from build123d import *

# Parameters (mm, degrees)
SKETCH_1_W               = 80
SKETCH_1_H               = 40
EXTRUDE_1_DEPTH          = 500
EXTRUDE_1_2_DEPTH        = 500
SKETCH_2_W               = 340
SKETCH_2_H               = 40
EXTRUDE_2_DEPTH          = 40
SKETCH_3_W               = 340
SKETCH_3_H               = 40
EXTRUDE_3_DEPTH          = 40
CUT_EXTRUDE_1_DEPTH      = 1
CUT_EXTRUDE_1_DEPTH_BACK = 161
SKETCH_5_W               = 40
SKETCH_5_H               = 200
EXTRUDE_4_DEPTH          = 40
SKETCH_6_W               = 40
SKETCH_6_H               = 200
EXTRUDE_5_DEPTH          = 40


with BuildPart() as part:
    # Sketch 1 → Extrude 1 (new body)
    with BuildSketch(Plane(origin=(0, 0, 0), x_dir=(1, 0, 0), z_dir=(0, 1, 0))):
        with Locations((40, -20)):
            Rectangle(SKETCH_1_W, SKETCH_1_H)
    extrude(amount=EXTRUDE_1_DEPTH)



with BuildPart() as body_2:
    # Sketch 1 → Extrude 1 2 (new body)
    with BuildSketch(Plane(origin=(0, 0, 0), x_dir=(1, 0, 0), z_dir=(0, 1, 0))):
        with Locations((40, 80)):
            Rectangle(SKETCH_1_W, SKETCH_1_H)
    extrude(amount=EXTRUDE_1_2_DEPTH)


with BuildPart() as part_1:
    add(part.part)

    add(body_2.part)  # Extrude 2 merges body 2
    # Sketch 2 → Extrude 2 (add)
    with BuildSketch(Plane(origin=(80, 0, 0), x_dir=(0, 0, -1), z_dir=(1, 0, 0))):
        with Locations((30, 480)):
            Rectangle(SKETCH_2_W, SKETCH_2_H)
    extrude(amount=EXTRUDE_2_DEPTH)

    # Sketch 3 → Extrude 3 (add)
    with BuildSketch(Plane.ZY):
        with Locations((-30, 480)):
            Rectangle(SKETCH_3_W, SKETCH_3_H)
    extrude(amount=EXTRUDE_3_DEPTH)

    # Sketch 4 → Cut-Extrude 1 (cut, two sides)
    with BuildSketch(Plane.ZY.offset(40)) as cut_extrude_1_sk:
        Polygon((140, 460), (100, 500), (140, 500), align=None)
        Polygon((-200, 460), (-160, 500), (-200, 500), align=None)
    extrude(amount=CUT_EXTRUDE_1_DEPTH, mode=Mode.SUBTRACT)
    extrude(cut_extrude_1_sk.sketch, amount=-CUT_EXTRUDE_1_DEPTH_BACK, mode=Mode.SUBTRACT)

    # Sketch 5 → Extrude 4 (add)
    with BuildSketch(Plane(origin=(0, 300, 300), x_dir=(1, 0, 0), z_dir=(0, 0.707106781, 0.707106781))):
        with Locations((-20, 222.842712475)):
            Rectangle(SKETCH_5_W, SKETCH_5_H)
        with Locations((100, 222.842712475)):
            Rectangle(SKETCH_5_W, SKETCH_5_H)
    extrude(amount=EXTRUDE_4_DEPTH)

    # Sketch 6 → Extrude 5 (add)
    with BuildSketch(Plane(origin=(0, 330, -330), x_dir=(1, 0, 0), z_dir=(0, 0.707106781, -0.707106781))):
        with Locations((100, -180.416305603)):
            Rectangle(SKETCH_6_W, SKETCH_6_H)
        with Locations((-20, -180.416305603)):
            Rectangle(SKETCH_6_W, SKETCH_6_H)
    extrude(amount=EXTRUDE_5_DEPTH)


solid = part_1.part
Design review of the part built by this model. Coordinates are the model's own, in mm. A direction names the side the tool comes from. Coordinates: 2 decimals unless noted, no trailing zeros. Loops run counter-clockwise (first coordinate to the right, second up) from the corner with the lowest first, then second, coordinate; pieces in that order, holes last. Notation, with made-up numbers: M 33,58 L 67,58 A13 cw 67,65 Z; hole C 19,87 d2. An arc over 180 degrees is marked long. Answer as CSV lines item,"result".
Item 1: Add section B-B on x = 8.5. State the section outline as (y, z) points, plus the area to 3 significant figures.
Answer list:
outline,"M 0,-100 L 500,-100 L 500,-60 L 0,-60 Z; M 0,0 L 500,0 L 500,40 L 0,40 Z"
area,"40,000 mm²"
Item 2: The part is to be moulded in two halves that separate along X. For faces 1 (the face through (99.72, 400.807, -287.081)), 2 (the face through (120, 475, -29)), 3 (the face through (80, 480, -30)), say which applies: pulls with the +X half, pulls with the -X half, needs draft (parallel to the pull), parting line crosses it, or undercut.
Answer list:
face 1,"needs draft"
face 2,"pulls with the +X half"
face 3,"undercut"
Item 3: Add section C-C on y = 434. State the section outline as (x, z) points, plus the area to 3 significant figures.
Answer list:
outline,"M -40,-282.57 L 0,-282.57 L 0,-226 L -40,-226 Z; M -40,166 L 0,166 L 0,222.57 L -40,222.57 Z; M 0,-100 L 80,-100 L 80,-60 L 0,-60 Z; M 0,0 L 80,0 L 80,40 L 0,40 Z; M 80,-282.57 L 120,-282.57 L 120,-226 L 80,-226 Z; M 80,166 L 120,166 L 120,222.57 L 80,222.57 Z"
area,"15,500 mm²"
Item 4: For P1, Ø10, axis at x = 13, y = 275, coming from the +Z side; P2, Ø12, axis at x = 84.5, z = -106.5, coming from the -Y side; P3, Ø12, axis at x = 62.5, y = 424, coming from the -Z side, all flat-tipped, find the tip position at first contact; note any pin that passes through.
Answer list:
P1,"z = 40"
P2,"y = 460"
P3,"z = -100"
Item 5: Add section A-A on z = -109. State the section outline as (x, y) points, plus the area to 3 significant figures.
Answer list:
outline,"M -40,460 L 0,460 L 0,500 L -40,500 Z; M 80,460 L 120,460 L 120,500 L 80,500 Z"
area,"3,200 mm²"
Item 6: Add section D-D on z = 25.5. State the section outline as (x, y) points.
Answer list:
outline,"M -40,460 L 0,460 L 0,0 L 80,0 L 80,460 L 120,460 L 120,500 L -40,500 Z"
Item 7: Machinability: for faces 4 (the face through (80, 481, -191)), 5 (the face through (99.72, 542.23, 85.66)), 6 (the face through (0, 480, -30)), 7 (the face through (-20, 423, -237)), which of the approach directions +Z, -Z, +X, -X, +Y, -Y give a long, thin tool a straight path to every point of the face, cutting with its end or side? Answer none if there is none.
Answer list:
face 4,"-Z, +Y, -Y"
face 5,"+X, -X, +Y"
face 6,"+Y, -Y"
face 7,"+X, -X, -Y"
Item 8: For probe 1 along Z at (x, y) = (45, 63); probe 2 along X at (y, z) = (491.5, -43); probe 3 along X at (y, z) = (230.5, -69.5), list the stretches that pass through material, from the lowest coordinate up.
Answer list:
probe 1,"-100 to -60, 0 to 40"
probe 2,"-40 to 0, 80 to 120"
probe 3,"0 to 80"
